from build123d import *

# Parameters (mm, degrees)
SKETCH1_R           = 1.47
BOSS_EXTRUDE1_DEPTH = 1.5875
SKETCH2_W           = 40.7
SKETCH2_H           = 19.685
CUT_EXTRUDE1_DEPTH  = 107.113527059


with BuildPart() as part:
    # Sketch1 → Boss-Extrude1 (new, symmetric)
    with BuildSketch(Plane.XY):
        Polygon((-12.5, 75), (-71.825, 75), (-71.825, 12.5), (-75, 12.5), (-75, -12.5), (-71.825, -12.5), (-71.825, -75), (-12.5, -75), (-12.5, -71.825), (-1.47, -71.825), (-1.47, -68.125), (-3.25, -68.125), (-3.25, -65.525), (-1.47, -65.525), (-1.47, -61.825), (1.47, -61.825), (1.47, -65.525), (3.25, -65.525), (3.25, -68.125), (1.47, -68.125), (1.47, -71.825), (12.5, -71.825), (12.5, -75), (71.825, -75), (71.825, -12.5), (75, -12.5), (75, 12.5), (71.825, 12.5), (71.825, 75), (12.5, 75), (12.5, 71.825), (1.47, 71.825), (1.47, 68.125), (3.25, 68.125), (3.25, 65.525), (1.47, 65.525), (1.47, 61.825), (-1.47, 61.825), (-1.47, 65.525), (-3.25, 65.525), (-3.25, 68.125), (-1.47, 68.125), (-1.47, 71.825), (-12.5, 71.825), align=None)
        with Locations((-73.4125, 0)):
            Circle(SKETCH1_R, mode=Mode.SUBTRACT)
        with Locations(Location((73.4125, 0, 0), (0, 0, 180))):
            Circle(SKETCH1_R, mode=Mode.SUBTRACT)
    extrude(amount=BOSS_EXTRUDE1_DEPTH, both=True)

    # Sketch2 → Cut-Extrude1 (cut, through all)
    with BuildSketch(Plane.XY.offset(1.5875)):
        with Locations((10.5075, 0)):
            Rectangle(SKETCH2_W, SKETCH2_H)
    extrude(amount=-CUT_EXTRUDE1_DEPTH, mode=Mode.SUBTRACT)


solid = part.part
Design review of the part built by this model. Coordinates are the model's own, in mm. Round coordinates to 2 decimals unless told otherwise and drop trailing zeros. Write each loop counter-clockwise with the first axis right and the second up, starting at its lowest first coordinate (ties: lowest second). Pieces come first, ordered by that corner, then holes. Notation, with made-up numbers: M 66,-14 L 92,-14 A30 ccw 92,17 Z; hole C 82.5,49 d4. An arc over 180 degrees is marked long. One line per item, written item: value. Start each with the question number.
1. To check wall thickness, follow probe 1 along Y at (x, z) = (24, 0.75); probe 2 along Y at (x, z) = (0, -0.75) (1 decimal); probe 3 along X at (y, z) = (-35.5, -0.8) (3 decimals). State the ranges of each line that lie inside material, in increasing order. Write a range as from..to.
2. Clearance check with flat-ended pins moving along their axes: P1, Ø1.6, axis at y = -63.5, z = 0.5, coming from the -X side (3 decimals); P2, Ø1, axis at y = 69.5, z = 0.5, coming from the +X side (3 decimals); P3, Ø1, axis at x = 73.5, z = 0.5, coming from the +Y side. State where each tip first meets the part, or that it passes through.
3. Take a section at B-B on y = -26. State the section outline as (x, z) points (1 decimal), then the cut area to 3 significant figures.
4. Take a section at A-A on z = 0.6. State how many separate pieces and enclosed holes the cut face has, then the cut area to 3 significant figures.
Computed:
1. probe 1: y = -75..-9.84, 9.84..75
1. probe 2: y = -61.8..-9.8, 9.8..61.8
1. probe 3: x = -71.825..71.825
2. P1: stops at x = -71.825
2. P2: stops at x = 71.825
2. P3: stops at y = 12.5
3. outline: M -71.8,-1.6 L 71.8,-1.6 L 71.8,1.6 L -71.8,1.6 Z
3. area: 456 mm²
4. separate pieces: 1
4. enclosed holes: 3
4. area: 20,700 mm²
